The model under review builds one solid part; all positions refer to its coordinate system, in mm. Give positions to 0.01 mm unless a question says otherwise; leave off trailing zeros. Order: outer loops, then holes, each group sorted by start corner. A loop starts at its lowest first (then second) coordinate and runs counter-clockwise, first axis right, second up. Notation, with made-up numbers: (57.5, -27) - (103.5, -27) arc R7 ccw to (103.5, -22) - close; hole circle Ø3 at (31.5, -12). An arc over 180 degrees is marked (long way). Write item = value, one per line. Start each with the question number.
1. Mouldability with a two-part tool opening along Z and no side actions: class faces 1 (the cylindrical face through (29.9, 0, 94.9)), 2 (the flat face through (24, -1.5, -24)), 3 (the cylindrical face through (-31.24, -0.02, -6.94)) as pulls with the +Z half, pulls with the -Z half, needs draft (parallel to the pull), parting line crosses it, or undercut.
2. For P1, Ø1.5, axis at y = -0.5, z = 39, coming from the +X side, flat-tipped, find the tip position at first contact; note if it passes through.
3. We need section A-A, the plane y = -0.4. State how many separate pieces and enclosed holes the cut face has, and give its area (3 significant figures).
4. We need section B-B, the plane z = -86. Give the boundary of the cut face in (x, y), and give its area (3 significant figures).
5. Wall thickness on probe 1 along Z at (x, y) = (-5, -0.25); probe 2 along X at (y, z) = (-0.8, 0.5); probe 3 along X at (y, z) = (-1, -14.5): over which ranges is each line inside the solid? List them lowest first.
6. We need section C-C, the plane x = -36. Give the boundary of the cut face in (y, z).
from build123d import *

# Parameters (mm, degrees)
SKETCH1_R                     = 99.5
SKETCH1_R_2                   = 32
BASE_DEPTH                    = 1.5
SKETCH2_R                     = 2
STRUCTURAL_HOLE_DEPTH         = 141.746225527
STRUCTURAL_HOLE_PATTERN_COUNT = 8


with BuildPart() as part:
    # Sketch1 → Base (new, symmetric)
    with BuildSketch(Plane(origin=(0, 0, 0), x_dir=(1, 0, 0), z_dir=(0, 1, 0))):
        with Locations(Location((0, 0, 0), (0, 0, 270))):
            Circle(SKETCH1_R)
        with Locations(Location((0, 0, 0), (0, 0, 270))):
            Circle(SKETCH1_R_2, mode=Mode.SUBTRACT)
    extrude(amount=BASE_DEPTH, both=True)

    # Sketch2 → Structural Hole (cut, through all)
    with BuildSketch(Plane(origin=(0, 1.5, 0), x_dir=(1, 0, 0), z_dir=(0, 1, 0))):
        with Locations(Location((0, 94.5, 0), (0, 0, 270))):
            Circle(SKETCH2_R)
    structural_hole = extrude(amount=-STRUCTURAL_HOLE_DEPTH, mode=Mode.SUBTRACT)

    # Structural Hole Pattern: Structural Hole ×8 about axis
    structural_hole_pattern_axis = Axis((0, 0, 0), (0, 1, 0))
    for i in range(1, STRUCTURAL_HOLE_PATTERN_COUNT):
        add(structural_hole.rotate(structural_hole_pattern_axis, i * 360 / STRUCTURAL_HOLE_PATTERN_COUNT), mode=Mode.SUBTRACT)


solid = part.part
Model answer:
q1.face_1 = parting line crosses it
q1.face_2 = needs draft
q1.face_3 = undercut
q2.P1 = 91.85
q3.separate_pieces = 1
q3.enclosed_holes = 9
q3.area = 27,800 mm2
q4.outline = (-50.04, -1.5) - (50.04, -1.5) - (50.04, 1.5) - (-50.04, 1.5) - close
q4.area = 300 mm2
q5.probe_1 = -99.37 to -31.61, 31.61 to 99.37
q5.probe_2 = -99.5 to -96.44, -92.56 to -32, 32 to 92.56, 96.44 to 99.5
q5.probe_3 = -98.44 to -28.53, 28.53 to 98.44
q6.outline = (-1.5, -92.76) - (1.5, -92.76) - (1.5, 92.76) - (-1.5, 92.76) - close
